Build history of the part. All positions in model axes, mm. A direction names the side the tool comes from. Give positions to 0.01 mm unless a question says otherwise; leave off trailing zeros. Loops run counter-clockwise (first coordinate to the right, second up) from the corner with the lowest first, then second, coordinate; pieces in that order, holes last. Notation, with made-up numbers: (-20.75, 52.25) -> (3.25, 52.25) arc R28 ccw to (3.25, 88.25) -> close; hole circle Ø5 at (30, 51). An arc over 180 degrees is marked (long way). One line per question, with ' | ' between items. Start each with the question number.
(1) Slice it at D-D, the plane x = -5. Write the cut outline in (y, z) (3 decimals), then the cut area to 3 significant figures.
(2) 3-axis set-ups, long thin cutter, end or side, ignore diameter. For faces 1 (the face through (0.67, -3.44, 55.46)), 2 (the face through (-3, 0, 46)), 3 (the face through (1.321, 3.775, 55.465)), 4 (the face through (-3, 0, 55)): which of +Z, -Z, +X, -X, +Y, -Y reach the whole face in a straight line?
(3) Drill centre lines: L1, parallel to Z at x = -0.75, y = -2.75; L2, parallel to Z at x = -6, y = 2.5; L3, parallel to Y at x = 0.25, z = 28.5. Where is each one in solid material? Low to high. Write a range as from..to.
(4) Slice it at C-C, the plane z = 33. Write the cut outline in (x, y), then the cut area to 3 significant figures.
(5) Mould opens along Y. For faces 5 (the face through (3.408, -0.764, 55.465)), 6 (the face through (-1, 2, 53)), 7 (the face through (1.31, -3.78, 55.46)), 8 (the face through (3.51, 1.92, 55.46)) say: pulls with the +Y half, pulls with the -Y half, needs draft (parallel to the pull), parting line crosses it, or undercut.
(6) Slice it at A-A, the plane x = 0. Write the cut outline in (y, z), then the cut area to 3 significant figures.
(7) Flat gauge pins, fed straight in: pin 1 Ø3 at (x, y) = (-5, -3.5) entering from +Z; pin 2 Ø1.5 at (x, z) = (-4, 30.5) entering from -Y; pin 3 Ø4 at (y, z) = (6, 45) entering from -X. Where does each tip first touch, or does it go through?
```python
from build123d import *

# Parameters (mm, degrees)
ESBO_O1_R                = 8
RESSALTO_EXTRUS_O1_DEPTH = 45
ESBO_O2_R                = 3
RESSALTO_EXTRUS_O2_DEPTH = 3
ESBO_O3_R                = 2
RESSALTO_EXTRUS_O3_DEPTH = 5
ESBO_O4_R                = 4
RESSALTO_EXTRUS_O4_DEPTH = 5
ESBO_O5_R                = 2
RESSALTO_EXTRUS_O5_DEPTH = 1
CORTE_EXTRUS_O11_START   = -5
CORTE_EXTRUS_O11_DEPTH   = 5


# Read off the part's stored shape, not the designer's step: Corte-extrusão11
with BuildPart() as part:
    # Esboço1 → Ressalto-extrusão1 (new body)
    with BuildSketch(Plane.XY):
        with Locations(Location((0, 0, 0), (0, 0, 180))):
            Circle(ESBO_O1_R)
    extrude(amount=RESSALTO_EXTRUS_O1_DEPTH)

    # Esboço2 → Ressalto-extrusão2 (add)
    with BuildSketch(Plane.XY.offset(45)):
        Circle(ESBO_O2_R)
    extrude(amount=RESSALTO_EXTRUS_O2_DEPTH)

    # Esboço3 → Ressalto-extrusão3 (add)
    with BuildSketch(Plane.XY.offset(48)):
        Circle(ESBO_O3_R)
    extrude(amount=RESSALTO_EXTRUS_O3_DEPTH)

    # Esboço4 → Ressalto-extrusão4 (add)
    with BuildSketch(Plane.XY.offset(53)):
        Circle(ESBO_O4_R)
    extrude(amount=RESSALTO_EXTRUS_O4_DEPTH)

    # Esboço5 → Ressalto-extrusão5 (add)
    with BuildSketch(Plane.XY.offset(58)):
        Circle(ESBO_O5_R)
    extrude(amount=RESSALTO_EXTRUS_O5_DEPTH)

    # Corte-extrusão11 outline → Corte-extrusão11 (cut)
    with BuildSketch(Plane.XY.offset(58).offset(CORTE_EXTRUS_O11_START)):
        with BuildLine():
            ThreePointArc((-0.572247027, 2.944916525), (3.275e-06, 3), (0.572253456, 2.944915276))
            Line((0.572253456, 2.944915276), (0.763004609, 3.926553701))
            ThreePointArc((0.763004609, 3.926553701), (4.366e-06, 4), (-0.762996037, 3.926555367))
            Line((-0.762996037, 3.926555367), (-0.572247027, 2.944916525))
        make_face()
        with BuildLine():
            ThreePointArc((3.037246914, 2.602908216), (2.483346926, 3.135759564), (1.837759325, 3.552835581))
            Line((1.837759325, 3.552835581), (1.376093618, 2.660323526))
            ThreePointArc((1.376093618, 2.660323526), (1.780577016, 2.408422803), (2.139992834, 2.095563308))
            Line((2.139992834, 2.095563308), (3.037246914, 2.602908216))
        make_face()
        with BuildLine():
            Line((-1.376093618, 2.660323526), (-1.837759325, 3.552835581))
            ThreePointArc((-1.837759325, 3.552835581), (-2.483346926, 3.135759564), (-3.037246914, 2.602908216))
            Line((-3.037246914, 2.602908216), (-2.139992834, 2.095563308))
            ThreePointArc((-2.139992834, 2.095563308), (-1.780577016, 2.408422803), (-1.376093618, 2.660323526))
        make_face()
        with BuildLine():
            ThreePointArc((3.898015048, -0.897484644), (3.997519889, 0.140835844), (3.825190717, 1.169579401))
            Line((3.825190717, 1.169579401), (2.873235611, 0.857757981))
            ThreePointArc((2.873235611, 0.857757981), (2.996308475, 0.115616418), (2.93078938, -0.633802208))
            Line((2.93078938, -0.633802208), (3.898015048, -0.897484644))
        make_face()
        with BuildLine():
            Line((-2.873235611, 0.857757981), (-3.825190717, 1.169579401))
            ThreePointArc((-3.825190717, 1.169579401), (-3.997519889, 0.140835844), (-3.898015048, -0.897484644))
            Line((-3.898015048, -0.897484644), (-2.93078938, -0.633802208))
            ThreePointArc((-2.93078938, -0.633802208), (-2.996308475, 0.115616418), (-2.873235611, 0.857757981))
        make_face()
        with BuildLine():
            Line((-2.139992834, -2.095563308), (-3.037246914, -2.602908216))
            ThreePointArc((-3.037246914, -2.602908216), (-2.483346926, -3.135759564), (-1.837759325, -3.552835581))
            Line((-1.837759325, -3.552835581), (-1.376093618, -2.660323526))
            ThreePointArc((-1.376093618, -2.660323526), (-1.780577016, -2.408422803), (-2.139992834, -2.095563308))
        make_face()
        with BuildLine():
            ThreePointArc((1.837759325, -3.552835581), (2.483346926, -3.135759564), (3.037246914, -2.602908216))
            Line((3.037246914, -2.602908216), (2.139992834, -2.095563308))
            ThreePointArc((2.139992834, -2.095563308), (1.780577016, -2.408422803), (1.376093618, -2.660323526))
            Line((1.376093618, -2.660323526), (1.837759325, -3.552835581))
        make_face()
        with BuildLine():
            Line((-0.572247027, -2.944916525), (-0.762996037, -3.926555367))
            ThreePointArc((-0.762996037, -3.926555367), (4.366e-06, -4), (0.763004609, -3.926553701))
            Line((0.763004609, -3.926553701), (0.572253456, -2.944915276))
            ThreePointArc((0.572253456, -2.944915276), (3.275e-06, -3), (-0.572247027, -2.944916525))
        make_face()
    extrude(amount=CORTE_EXTRUS_O11_DEPTH, mode=Mode.SUBTRACT)


solid = part.part
```
Final values:
1) outline: (-6.245, 0) -> (6.245, 0) -> (6.245, 45) -> (-6.245, 45) -> close | area: 562 mm2
2) face 1: +Z, -Y | face 2: none | face 3: +Z, +X, +Y | face 4: +Z, -X
3) L1: 0..48, 53..58 | L2: 0..45 | L3: -8..8
4) outline: circle Ø16 at (0, 0) | area: 201 mm2
5) face 5: undercut | face 6: needs draft | face 7: pulls with the -Y half | face 8: pulls with the +Y half
6) outline: (-8, 0) -> (8, 0) -> (8, 45) -> (3, 45) -> (3, 48) -> (2, 48) -> (2, 53) -> (3, 53) -> (3, 58) -> (2, 58) -> (2, 59) -> (-2, 59) -> (-2, 58) -> (-3, 58) -> (-3, 53) -> (-2, 53) -> (-2, 48) -> (-3, 48) -> (-3, 45) -> (-8, 45) -> close | area: 792 mm2
7) pin 1: z = 45 | pin 2: y = -7.31 | pin 3: x = -6.93
